Here's how the part is built. I have some questions about the finished solid (model axes, mm). Face numbers are marked on the shaded views. A direction names the side the tool comes from. Give positions to 0.01 mm unless a question says otherwise; leave off trailing zeros. Loops run counter-clockwise (first coordinate to the right, second up) from the corner with the lowest first, then second, coordinate; pieces in that order, holes last. Notation, with made-up numbers: M 62.5,-30 L 103.5,-30 A31 cw 103.5,-3 Z; hole C 7.5,68.25 d1. An arc over 180 degrees is marked long. Answer as CSV lines item,"result". Start each with the question number.
Item 1: I want a section at B-B on x = -6.5. List the corners of the cut face in (y, z) for me.
Item 2: For the marked faces 1 and 2, which set-ups out of +Z, -Z, +X, -X, +Y, -Y let a thin tool reach every point of the face, with its end or its side?
Item 3: Will these pins go through, and if not, where does the flat tip stop? P1, Ø3, axis at y = 5.5, z = 0, coming from the +X side (3 decimals); P2, Ø0.8, axis at x = 9.525, z = 2.54, coming from the +Y side; P3, Ø1.7, axis at x = 9.525, z = -2.54, coming from the +Y side; P4, Ø3, axis at y = 4.5, z = 1, coming from the -X side (3 decimals).
Item 4: If I drill on line 1 along Z through (x, y) = (8, 0.5); line 2 along X through (y, z) = (2.5, 6.75) (3 decimals); line 3 along X through (y, z) = (0.75, 0) (3 decimals), over which ranges is the centre line in solid material (lowest first)? Write a range as from..to.
Item 5: I want a section at A-A on z = 0. List the corners of the cut face in (x, y) for me (3 decimals).
Item 6: If we mould it in two halves opening along X, with no side actions, what happens to the marked faces 3, 4, 5 and 6? For each: released by +X, released by -X, zero draft, split by the parting line, or undercut.
Item 7: I want a section at D-D on y = 2. List the corners of the cut face in (x, z) for me (3 decimals), plus the area to 3 significant figures.
Item 8: I want a section at C-C on z = -6.35. List the corners of the cut face in (x, y) for me (3 decimals), plus the area to 3 significant figures.
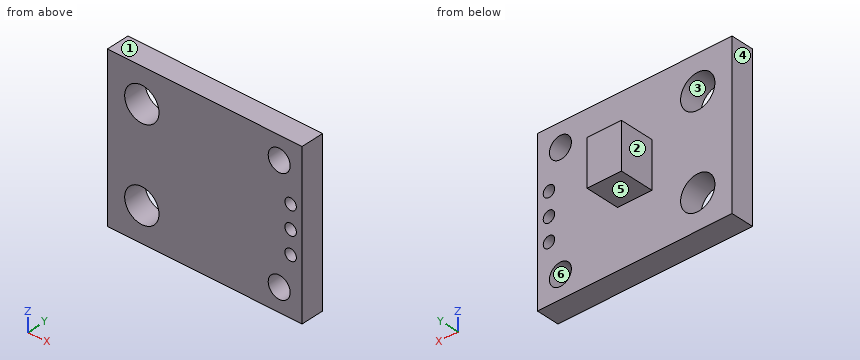
from build123d import *

# Parameters (mm, degrees)
SKETCH1_W                 = 21.59
SKETCH1_H                 = 17.78
BOSS_EXTRUDE1_DEPTH       = 2.54
SKETCH2_R                 = 1.905
SKETCH2_R_2               = 0.635
CUT_EXTRUDE1_DEPTH        = 15.213223596
SKETCH3_W                 = 3.81
SKETCH3_H                 = 5.08
BOSS_EXTRUDE2_DEPTH       = 3.81
F_2_CLEARANCE_HOLE1_D     = 2.4384
F_2_CLEARANCE_HOLE1_DEPTH = 6.35
F_2_CLEARANCE_HOLE1_TIP   = 0.732569267


with BuildPart() as part:
    # Sketch1 → Boss-Extrude1 (new body)
    with BuildSketch(Plane(origin=(0, 0, 0), x_dir=(1, 0, 0), z_dir=(0, 1, 0))):
        Rectangle(SKETCH1_W, SKETCH1_H)
    extrude(amount=BOSS_EXTRUDE1_DEPTH)

    # Sketch2 → Cut-Extrude1 (cut, through all)
    with BuildSketch(Plane(origin=(0, 2.54, 0), x_dir=(1, 0, 0), z_dir=(0, 1, 0))):
        with Locations(Location((-6.985, 5.08, 0), (0, 0, 270))):
            Circle(SKETCH2_R)
        with Locations(Location((-6.985, -5.08, 0), (0, 0, 270))):
            Circle(SKETCH2_R)
        with Locations(Location((9.525, 2.54, 0), (0, 0, 270))):
            Circle(SKETCH2_R_2)
        with Locations(Location((9.525, 0, 0), (0, 0, 270))):
            Circle(SKETCH2_R_2)
        with Locations(Location((9.525, -2.54, 0), (0, 0, 270))):
            Circle(SKETCH2_R_2)
    extrude(amount=-CUT_EXTRUDE1_DEPTH, mode=Mode.SUBTRACT)

    # Sketch3 → Boss-Extrude2 (add)
    with BuildSketch(Plane(origin=(0, 2.54, 0), x_dir=(1, 0, 0), z_dir=(0, 1, 0))):
        Rectangle(SKETCH3_W, SKETCH3_H)
    extrude(amount=BOSS_EXTRUDE2_DEPTH)

    # #2 Clearance Hole1
    with Locations(Plane(origin=(0, 2.54, 0), x_dir=(1, 0, 0), z_dir=(0, 1, 0))):
        with Locations((8.255, 6.35), (8.255, -6.35)):
            Hole(F_2_CLEARANCE_HOLE1_D / 2, depth=F_2_CLEARANCE_HOLE1_DEPTH)
            with Locations((0, 0, -(F_2_CLEARANCE_HOLE1_DEPTH + F_2_CLEARANCE_HOLE1_TIP / 2))):  # 118° drill point
                Cone(0, F_2_CLEARANCE_HOLE1_D / 2, F_2_CLEARANCE_HOLE1_TIP, mode=Mode.SUBTRACT)


solid = part.part
Result:
1,outline,"M 0,-8.89 L 2.54,-8.89 L 2.54,-6.92 L 0,-6.92 Z; M 0,-3.24 L 2.54,-3.24 L 2.54,3.24 L 0,3.24 Z; M 0,6.92 L 2.54,6.92 L 2.54,8.89 L 0,8.89 Z"
2,face 1,"+Z, +X, -X, +Y, -Y"
2,face 2,"+Z, -Z, -X, +Y"
3,P1,"x = 1.905"
3,P2,"through"
3,P3,"y = 2.54"
3,P4,"x = -1.905"
4,line 1,"-8.89..-7.54, -5.16..5.16, 7.54..8.89"
4,line 2,"-10.795..-7.902, -6.068..7.103, 9.407..10.795"
4,line 3,"-10.795..8.89, 10.16..10.795"
5,outline,"M -10.795,0 L 8.89,0 L 8.89,2.54 L 1.905,2.54 L 1.905,6.35 L -1.905,6.35 L -1.905,2.54 L -10.795,2.54 Z; M 10.16,0 L 10.795,0 L 10.795,2.54 L 10.16,2.54 Z"
6,face 3,"undercut"
6,face 4,"released by -X"
6,face 5,"zero draft"
6,face 6,"undercut"
7,outline,"M -10.795,-8.89 L 10.795,-8.89 L 10.795,8.89 L -10.795,8.89 Z; hole C -6.985,-5.08 d3.81; hole C -6.985,5.08 d3.81; hole C 8.255,-6.35 d2.438; hole C 8.255,6.35 d2.438; hole C 9.525,-2.54 d1.27; hole C 9.525,0 d1.27; hole C 9.525,2.54 d1.27"
7,area,"348 mm^2"
8,outline,"M -10.795,0 L -8.405,0 L -8.405,2.54 L -10.795,2.54 Z; M -5.565,0 L 7.036,0 L 7.036,2.54 L -5.565,2.54 Z; M 9.474,0 L 10.795,0 L 10.795,2.54 L 9.474,2.54 Z"
8,area,"41.4 mm^2"
